Autodesk Inventor part; units mm, degrees
ref_plane "YZ Plane" through (0, 0, 0) normal (1, 0, 0) x (0, 1, 0)
ref_plane "XZ Plane" through (0, 0, 0) normal (0, 1, 0) x (-1, 0, 0)
ref_plane "XY Plane" through (0, 0, 0) normal (0, 0, 1) x (1, 0, 0)
sketch "Эскиз1" plane through (0, 0, 0) normal (0, 0, 1) x (1, 0, 0)
  line L0 (0, 9) -> (0, -9) construction
  line L1 (0, -9) -> (10, -9)
  arc A0 (0, -2.25) -> (0, 4.25) centre (0, 1) ccw
  arc A1 (7.8648, 2.4648) -> (0, 9) centre (0, 1) ccw
  line L2 (7.8648, 2.4648) -> (10, -9)
  line L3 (0, 9) -> (0, 4.25)
  line L4 (0, -2.25) -> (0, -9)
  point P0 (0, 0)
  point P1 (0, 0)
  dimension "d0" = 18
  dimension "d1" = 10
  dimension "d2" = 3.25
  dimension "d3" = 10
extrude "Выдавливание1" add sketch "Эскиз1" along normal blind 1
mirror "Зеркальное отражение1" about plane through (0, 0, 0) normal (1, 0, 0) of "Выдавливание1"
properties part number "76. Стопор штуцера"
Input: part model. Units: mm. Frame: model coordinates. Coordinates: 2 decimals unless noted, no trailing zeros. Write each loop counter-clockwise with the first axis right and the second up, starting at its lowest first coordinate (ties: lowest second). Pieces come first, ordered by that corner, then holes. Notation, with made-up numbers: (7.25, 78.5) -> (16.25, 78.5) arc R22 cw to (16.25, 101.5) -> close; hole circle Ø3 at (67.25, -20.5). An arc over 180 degrees is marked (long way). Answer as a JSON object with one key per item and string values.
1. Material intervals for line 1 (Y direction, x = 0, z = 0.5); line 2 (X direction, y = -0.5, z = 0.45); line 3 (X direction, y = 1, z = 0.7), sorted ascending. Write a range as from..to.
Result set:
{"line 1": "y = -9..-2.25, 4.25..9", "line 2": "x = -8.42..-2.88, 2.88..8.42", "line 3": "x = -8.14..-3.25, 3.25..8.14"}
2. Mould query, pull axis X, two halves, no side actions, for faces 1 (the face through (8.917, -3.187, 0.493)), 2 (the face through (-8.947, -3.348, 0.493)), 3 (the face through (2.883, -0.5, 0.493)), 4 (the face through (2, -2, 1)). Classes: released by +X, released by -X, zero draft, split by the parting line, or undercut.
Result set:
{"face 1": "released by +X", "face 2": "released by -X", "face 3": "undercut", "face 4": "zero draft"}
3. Section A-A on y = 1. Return the cut outline in (x, z), then the cut area to 3 significant figures.
Result set:
{"outline": "(-8.14, 0) -> (-3.25, 0) -> (-3.25, 1) -> (-8.14, 1) -> close; (3.25, 0) -> (8.14, 0) -> (8.14, 1) -> (3.25, 1) -> close", "area": "9.78 mm2"}
4. Section B-B on z = 0.25. Return the cut outline in (x, y).
Result set:
{"outline": "(-10, -9) -> (10, -9) -> (7.86, 2.46) arc R8 ccw to (0, 9) arc R8 ccw to (-7.86, 2.46) -> close; hole circle Ø6.5 at (0, 1)"}
5. Section C-C on x = -6. Return the cut outline in (y, z), then the cut area to 3 significant figures.
Result set:
{"outline": "(-9, 0) -> (6.29, 0) -> (6.29, 1) -> (-9, 1) -> close", "area": "15.3 mm2"}
6. Section D-D on y = 7.75. Return the cut outline in (x, z), then the cut area to 3 significant figures.
Result set:
{"outline": "(-4.29, 0) -> (4.29, 0) -> (4.29, 1) -> (-4.29, 1) -> close", "area": "8.59 mm2"}
